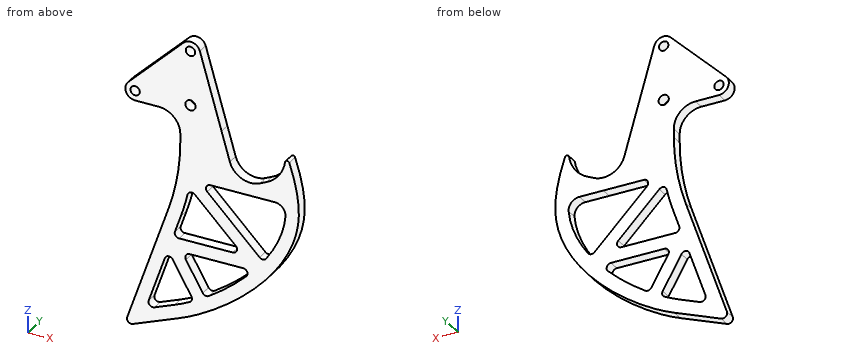
from build123d import *

# Parameters (mm, degrees)
SKETCH1_R           = 2.35
SKETCH1_R_2         = 2.15
BOSS_EXTRUDE1_DEPTH = 5
BOSS_EXTRUDE2_DEPTH = 5
FILLET9_START       = -1
FILLET9_DEPTH       = 7
FILLET10_R          = 10
FILLET11_R          = 10
FILLET12_R          = 2
FILLET13_R          = 100
CUT_EXTRUDE1_DEPTH  = 10
FILLET16_R          = 2
FILLET17_R          = 5


with BuildPart() as part:
    # Sketch1 → Boss-Extrude1 (new body)
    # profile 1 of 5: a face of its own
    with BuildSketch(Plane(origin=(0, 0, 0), x_dir=(1, 0, 0), z_dir=(0, 1, 0))):
        with BuildLine():
            Line((21.319657121, 32.633890732), (34.914273926, 26.294616806))
            ThreePointArc((34.914273926, 26.294616806), (41.225871687, 20.759494125), (43.575, 12.7))
            ThreePointArc((43.575, 12.7), (43.275555611, 9.717775204), (42.389178035, 6.854618472))
            add(Edge.make_bspline(
                [(42.389178035, 6.854618472), (44.342966782, 11.471936513), (48.441890724, 22.813367807), (54.26521217, 62.473053577), (15.464484864, 91.951031047), (-5, 100)],
                knots=[0, 0, 0, 0, 0.134757694, 0.296973126, 1, 1, 1, 1], degree=3))
            Line((-5, 100), (-4.618360102, 4.58315657))
            Line((-4.618360102, 4.58315657), (-4.499964006, -25.01799856))
            ThreePointArc((-4.499964006, -25.01799856), (-0.008999298, -20.500008999), (4.5, -25))
            ThreePointArc((4.5, -25), (4.455654175, -25.630195106), (4.323490724, -26.247969535))
            Line((4.323490724, -26.247969535), (14.266400512, 8.198446858))
            ThreePointArc((14.266400512, 8.198446858), (14.163364253, 16.859898449), (18.866215247, 24.134137424))
            Line((18.866215247, 24.134137424), (21.319657121, 32.633890732))
        make_face()
        with Locations(Location((0, 0, 0), (0, 0, 270))):
            Circle(SKETCH1_R, mode=Mode.SUBTRACT)
    # profile 2 of 5: a face of its own
    with BuildSketch(Plane(origin=(0, 0, 0), x_dir=(1, 0, 0), z_dir=(0, 1, 0))):
        with BuildLine():
            Line((14.266400512, 8.198446858), (18.866215247, 24.134137424))
            ThreePointArc((18.866215247, 24.134137424), (14.163364253, 16.859898449), (14.266400512, 8.198446858))
        make_face()
    # profile 3 of 5: a face of its own
    with BuildSketch(Plane(origin=(0, 0, 0), x_dir=(1, 0, 0), z_dir=(0, 1, 0))):
        with BuildLine():
            ThreePointArc((-3.156627288, -28.207133325), (1.140163698, -29.353162843), (4.323490724, -26.247969535))
            ThreePointArc((4.323490724, -26.247969535), (4.455654175, -25.630195106), (4.5, -25))
            ThreePointArc((4.5, -25), (-0.008999298, -20.500008999), (-4.499964006, -25.01799856))
            ThreePointArc((-4.499964006, -25.01799856), (-4.147106545, -26.746856406), (-3.156627288, -28.207133325))
        make_face()
        with Locations(Location((0, -25, 0), (0, 0, 270))):
            Circle(SKETCH1_R_2, mode=Mode.SUBTRACT)
    # profile 4 of 5: a face of its own
    with BuildSketch(Plane(origin=(0, 0, 0), x_dir=(1, 0, 0), z_dir=(0, 1, 0))):
        with BuildLine():
            Line((-4.499964006, -25.01799856), (-4.618360102, 4.58315657))
            Line((-4.618360102, 4.58315657), (-25.41799856, 4.499964006))
            ThreePointArc((-25.41799856, 4.499964006), (-22.224389312, 3.188337617), (-20.9, 0))
            ThreePointArc((-20.9, 0), (-23.661440653, -4.150591693), (-28.556627288, -3.207133325))
            Line((-28.556627288, -3.207133325), (-3.156627288, -28.207133325))
            ThreePointArc((-3.156627288, -28.207133325), (-4.147106545, -26.746856406), (-4.499964006, -25.01799856))
        make_face()
    # profile 5 of 5: a face of its own
    with BuildSketch(Plane(origin=(0, 0, 0), x_dir=(1, 0, 0), z_dir=(0, 1, 0))):
        with BuildLine():
            ThreePointArc((-20.9, 0), (-22.224389312, 3.188337617), (-25.41799856, 4.499964006))
            ThreePointArc((-25.41799856, 4.499964006), (-29.567661171, 1.69723315), (-28.556627288, -3.207133325))
            ThreePointArc((-28.556627288, -3.207133325), (-23.661440653, -4.150591693), (-20.9, 0))
        make_face()
        with Locations(Location((-25.4, 0, 0), (0, 0, 270))):
            Circle(SKETCH1_R_2, mode=Mode.SUBTRACT)
    extrude(amount=BOSS_EXTRUDE1_DEPTH)

    # Sketch2 → Boss-Extrude2 (add, through all)
    with BuildSketch(Plane(origin=(0, 5, 0), x_dir=(1, 0, 0), z_dir=(0, 1, 0))):
        Polygon((-5, 100), (-30.440224277, 110.005997059), (-4.740018717, 35), align=None)
    extrude(amount=-BOSS_EXTRUDE2_DEPTH)

    # Fillet9: read off the stored shape, not the designer's step
    # Fillet9 outline → Fillet9 (cut)
    with BuildSketch(Plane(origin=(0, 0, 0), x_dir=(1, 0, 0), z_dir=(0, 1, 0)).offset(FILLET9_START)):
        with BuildLine():
            add(Edge.make_bspline(
                [(42.389178035, 6.854618472), (43.427373548, 9.308148252), (44.439078816, 11.911072083), (45.365164545, 14.597488782)],
                knots=[0, 0, 0, 0, 0.07160694, 0.07160694, 0.07160694, 0.07160694], degree=3))
            ThreePointArc((45.365164545, 14.597488782), (44.323632558, 13.928027401), (43.429465164, 14.784433901))
            ThreePointArc((43.429465164, 14.784433901), (43.447567664, 10.748915407), (42.389178035, 6.854618472))
        make_face()
    extrude(amount=FILLET9_DEPTH, mode=Mode.SUBTRACT)

    # Fillet10
    fillet10_edges = [part.edges().sort_by_distance(p)[0] for p in [
        (21.319657121, 2.5, -32.633890732),
    ]]
    fillet(fillet10_edges, radius=FILLET10_R)

    # Fillet11
    fillet11_edges = [part.edges().sort_by_distance(p)[0] for p in [
        (-4.618360102, 2.5, -4.58315657),
    ]]
    fillet(fillet11_edges, radius=FILLET11_R)

    # Fillet12
    fillet12_edges = [part.edges().sort_by_distance(p)[0] for p in [
        (-30.440224277, 2.5, -110.005997059),
    ]]
    fillet(fillet12_edges, radius=FILLET12_R)

    # Fillet13
    fillet13_edges = [part.edges().sort_by_distance(p)[0] for p in [
        (-4.740018717, 2.5, -35),
    ]]
    fillet(fillet13_edges, radius=FILLET13_R)

    # Sketch3 → Cut-Extrude1 (cut)
    with BuildSketch(Plane(origin=(0, 5, 0), x_dir=(1, 0, 0), z_dir=(0, 1, 0))):
        with BuildLine():
            Line((-7.196124056, 94.416359688), (-20.556666638, 99.671248494))
            Line((-20.556666638, 99.671248494), (-10.34167973, 69.858830216))
            Line((-10.34167973, 69.858830216), (1.479992408, 90.33456699))
            add(Edge.make_bspline(
                [(1.479992408, 90.33456699), (1.28397872, 90.440564461), (0.569604437, 90.823664357), (-0.911069003, 91.59331249), (-2.926185163, 92.579659505), (-4.750200244, 93.404717974), (-6.168292078, 94.005080785), (-6.85002115, 94.280232561), (-7.196124056, 94.416359688)],
                knots=[0.899537877, 0.899537877, 0.899537877, 0.899537877, 0.905955438, 0.922989268, 0.948659512, 0.974329756, 0.987164878, 1, 1, 1, 1], degree=3))
        make_face()
        with BuildLine():
            add(Edge.make_bspline(
                [(28.891913577, 69.093470772), (28.667354165, 69.339735814), (26.185201557, 72.030266697), (22.009276054, 76.029258723), (16.240637184, 80.752486943), (11.640954059, 84.113026779), (8.44218135, 86.220773941), (6.886134042, 87.191294266), (6.670477462, 87.324750819)],
                knots=[0.599769047, 0.599769047, 0.599769047, 0.599769047, 0.608173487, 0.691957071, 0.743297559, 0.794638047, 0.837083391, 0.84392152, 0.84392152, 0.84392152, 0.84392152], degree=3))
            Line((6.670477462, 87.324750819), (-3.855356981, 69.093470772))
            Line((-3.855356981, 69.093470772), (28.891913577, 69.093470772))
        make_face()
        with BuildLine():
            Line((24.256703875, 63.093470772), (-8.023583375, 63.093470772))
            Line((-8.023583375, 63.093470772), (-4.396532038, 52.507928907))
            ThreePointArc((-4.396532038, 52.507928907), (-2.247165573, 45.44102658), (-0.595170682, 38.241596216))
            Line((-0.595170682, 38.241596216), (24.256703875, 63.093470772))
        make_face()
        with BuildLine():
            add(Edge.make_bspline(
                [(43.683908276, 34.631385763), (43.696866831, 34.851470147), (43.767861036, 36.240626578), (43.768636498, 39.331228462), (43.211809078, 43.755898325), (41.817266975, 48.782881707), (39.714268813, 53.778597693), (37.032666408, 58.583202787), (34.774401672, 61.875598877), (33.528556835, 63.529710734), (33.377122853, 63.728608376)],
                knots=[0.24062608, 0.24062608, 0.24062608, 0.24062608, 0.247043641, 0.281233166, 0.332573654, 0.383914142, 0.43525463, 0.486595118, 0.533806823, 0.540275717, 0.540275717, 0.540275717, 0.540275717], degree=3))
            Line((33.377122853, 63.728608376), (4.279900241, 34.631385764))
            Line((4.279900241, 34.631385764), (27.686110097, 34.631385764))
            Line((27.686110097, 34.631385764), (43.683908276, 34.631385763))
        make_face()
    extrude(amount=-CUT_EXTRUDE1_DEPTH, mode=Mode.SUBTRACT)

    # Fillet16
    fillet16_edges = [part.edges().sort_by_distance(p)[0] for p in [
        (33.377122853, 2.5, -63.728608376),
        (-20.556666638, 2.5, -99.671248494),
        (-10.34167973, 2.5, -69.858830216),
        (1.479992408, 2.5, -90.33456699),
        (6.670477462, 2.5, -87.324750819),
        (-3.855356981, 2.5, -69.093470772),
        (28.891913577, 2.5, -69.093470772),
        (-8.023583375, 2.5, -63.093470772),
        (-0.595170682, 2.5, -38.241596216),
        (24.256703875, 2.5, -63.093470772),
        (4.279900241, 2.5, -34.631385764),
    ]]
    fillet(fillet16_edges, radius=FILLET16_R)

    # Fillet17
    fillet17_edges = [part.edges().sort_by_distance(p)[0] for p in [
        (43.683908276, 2.5, -34.631385763),
    ]]
    fillet(fillet17_edges, radius=FILLET17_R)


solid = part.part
Design review of the part built by this model. Coordinates are the model's own, in mm. Give positions to 0.01 mm unless a question says otherwise; leave off trailing zeros. Order: outer loops, then holes, each group sorted by start corner. A loop starts at its lowest first (then second) coordinate and runs counter-clockwise, first axis right, second up.
1. For pin 1 Ø1 at (y, z) = (2.5, -74.5) entering from -X; pin 2 Ø2.5 at (x, y) = (19.5, 2.5) entering from -Z; pin 3 Ø5 at (x, z) = (0, 25) entering from +Y; pin 4 Ø2.5 at (x, y) = (35, 3.5) entering from -Z, all flat-tipped, find the tip position at first contact; note any pin that passes through.
Solution:
pin 1: stops at x = -18.45
pin 2: stops at z = -86.69
pin 3: stops at y = 5
pin 4: stops at z = -72.67
2. Add section B-B, the plane y = 2.65. State how many separate pieces and enclosed holes the cut face has, then the cut area to 3 significant figures.
Solution:
separate pieces: 1
enclosed holes: 7
area: 3,590 mm2
3. Add section A-A, the plane x = -21.5. State the section outline as (y, z) points, then the cut area to 3 significant figures.
Solution:
outline: (0, -106.49) - (5, -106.49) - (5, -83.91) - (0, -83.91) - close; (0, -4.52) - (5, -4.52) - (5, 10.15) - (0, 10.15) - close
area: 186 mm2
4. Add section D-D, the plane z = 13. State the section outline as (x, y) points.
Solution:
outline: (-18.61, 0) - (8.15, 0) - (8.15, 5) - (-18.61, 5) - close
5. To check wall thickness, follow L1, parallel to Z at x = 19.5, y = 2.8; L2, parallel to X at y = 2, z = -75; L3, parallel to X at y = 2.5, z = 0. State the ranges of each line that lie inside material, in increasing order.
Solution:
L1: z = -85.74 to -78.06, -69.09 to -63.09, -58.34 to -49.85, -34.63 to -24.37
L2: x = -18.45 to -12.1, -7.37 to -0.45, 22.99 to 31.58
L3: x = -29.9 to -27.55, -23.25 to -2.35, 2.35 to 11.9
